Could you check a few things on this model? Use its own coordinates, in mm. A direction names the side the tool comes from. Give positions to 0.01 mm unless a question says otherwise; leave off trailing zeros. Loops run counter-clockwise (first coordinate to the right, second up) from the corner with the lowest first, then second, coordinate; pieces in that order, holes last. Notation, with made-up numbers: M 55.5,44.5 L 69.5,44.5 A24 ccw 69.5,60.5 Z; hole C 17,27 d7. An arc over 180 degrees is marked long. Use a Markdown table: item, result. Add a question column.
1) Suppose I cut it at C-C on y = 13.75. List the corners of the cut face in (x, z) for me.
2) Which directions (+Z, -Z, +X, -X, +Y, -Y) give clear straight access to the entire face, cutting with the end or side of a thin tool? Please do faces 4 (the flat face through (8, 9, 8)), 5 (the cylindrical face through (-12.04, 5.53, 20.46)), 6 (the flat face through (5, 11, 0)).
3) Suppose I cut it at B-B on z = 0. Count the separate pieces of the cut face and the enclosed holes in it, and give its area (3 significant figures).
4) Suppose I cut it at D-D on x = 26. List the corners of the cut face in (y, z) for me, and give its area (3 significant figures).
5) We'd pull the mould along X, two halves only. Please class faces 1 (the flat face through (-8, 11, 20)), 2 (the cylindrical face through (-32.19, 2.54, -32.84)), 3 (the flat face through (11, 8, 28)): +X half, -X half, draft (parallel to the pull), parting line (faces both ways), or undercut.
6) Will these pins go through, and if not, where does the flat tip stop? pin 1 Ø7 at (x, z) = (34, -34) entering from +Y; pin 2 Ø4 at (y, z) = (9, -10) entering from +X; pin 3 Ø3.5 at (y, z) = (9, -9.5) entering from -X.
7) Suppose I cut it at A-A on y = 1.25. List the corners of the cut face in (x, z) for me.
8) If I drill on line 1 along X through (y, z) = (11, 6.5); line 2 along Z through (x, y) = (5.8, 9); line 3 along X through (y, z) = (10.5, 18), over which ranges is the centre line in solid material (lowest first)? Write a range as [from, to].
```python
from build123d import *

# Parameters (mm, degrees)
SKETCH1_W           = 88
SKETCH1_H           = 88
BOSS_EXTRUDE1_DEPTH = 5
FILLET1_R           = 10
SKETCH2_R           = 2.15
CUT_EXTRUDE1_DEPTH  = 63.42595614
SKETCH3_W           = 4
SKETCH3_H           = 50
BOSS_EXTRUDE2_DEPTH = 10
CHAMFER1_SIZE       = 10
SKETCH4_R           = 1.5
CUT_EXTRUDE2_DEPTH  = 65.007812023
SKETCH5_R           = 3.5
CUT_EXTRUDE3_DEPTH  = 36
CUT_EXTRUDE4_START  = -36
SKETCH6_R           = 3.5
CUT_EXTRUDE4_DEPTH  = 36
LPATTERN2_COUNT     = 5
LPATTERN2_PITCH     = 10
CHAMFER2_SIZE       = 6


with BuildPart() as part:
    # Sketch1 → Boss-Extrude1 (new body)
    with BuildSketch(Plane(origin=(0, 0, 0), x_dir=(1, 0, 0), z_dir=(0, 1, 0))):
        Rectangle(SKETCH1_W, SKETCH1_H)
    extrude(amount=BOSS_EXTRUDE1_DEPTH)

    # Fillet1
    fillet1_edges = [part.edges().sort_by_distance(p)[0] for p in [
        (-44, 2.5, -44),
        (44, 2.5, -44),
        (44, 2.5, 44),
        (-44, 2.5, 44),
    ]]
    fillet(fillet1_edges, radius=FILLET1_R)

    # Sketch2 → Cut-Extrude1 (cut, through all)
    with BuildSketch(Plane(origin=(0, 5, 0), x_dir=(1, 0, 0), z_dir=(0, 1, 0))):
        with Locations(Location((34, 34, 0), (0, 0, 270))):
            Circle(SKETCH2_R)
        with Locations(Location((34, -34, 0), (0, 0, 270))):
            Circle(SKETCH2_R)
        with Locations(Location((-34, -34, 0), (0, 0, 270))):
            Circle(SKETCH2_R)
        with Locations(Location((-34, 34, 0), (0, 0, 270))):
            Circle(SKETCH2_R)
    extrude(amount=-CUT_EXTRUDE1_DEPTH, mode=Mode.SUBTRACT)

    # Sketch3 → Boss-Extrude2 (add)
    with BuildSketch(Plane(origin=(0, 5, 0), x_dir=(1, 0, 0), z_dir=(0, 1, 0))):
        with Locations((-7, 0)):
            Rectangle(SKETCH3_W, SKETCH3_H)
        with Locations((7, 0)):
            Rectangle(SKETCH3_W, SKETCH3_H)
    extrude(amount=BOSS_EXTRUDE2_DEPTH)

    # Chamfer1
    chamfer1_edges = [part.edges().sort_by_distance(p)[0] for p in [
        (9, 5, 0),
        (-9, 5, 0),
    ]]
    chamfer(chamfer1_edges, length=CHAMFER1_SIZE - 0.0001)  # a hair under: the kernel refuses the full size

    # Sketch4 → Cut-Extrude2 (cut, symmetric)
    with BuildSketch(Plane(origin=(0, 0, 0), x_dir=(0, 0, -1), z_dir=(1, 0, 0))):
        with Locations(Location((-20, 9, 0), (0, 0, 90))):
            Circle(SKETCH4_R)
    cut_extrude2 = extrude(amount=CUT_EXTRUDE2_DEPTH, both=True, mode=Mode.SUBTRACT)

    # Sketch5 → Cut-Extrude3 (cut)
    with BuildSketch(Plane(origin=(44, 0, 0), x_dir=(0, 0, -1), z_dir=(1, 0, 0))):
        with Locations((-20, 9)):
            Circle(SKETCH5_R)
    cut_extrude3 = extrude(amount=-CUT_EXTRUDE3_DEPTH, mode=Mode.SUBTRACT)

    # Sketch6 → Cut-Extrude4 (cut)
    with BuildSketch(Plane.ZY.offset(44).offset(CUT_EXTRUDE4_START)):
        with Locations(Location((20, 9, 0), (0, 0, 180))):
            Circle(SKETCH6_R)
    cut_extrude4 = extrude(amount=CUT_EXTRUDE4_DEPTH, mode=Mode.SUBTRACT)

    # LPattern2: Cut-Extrude2, Cut-Extrude3, Cut-Extrude4 ×5
    with Locations(*[(0, 0, -i * LPATTERN2_PITCH) for i in range(1, LPATTERN2_COUNT)]):
        add(cut_extrude2, mode=Mode.SUBTRACT)
        add(cut_extrude3, mode=Mode.SUBTRACT)
        add(cut_extrude4, mode=Mode.SUBTRACT)

    # Chamfer2
    chamfer2_edges = [part.edges().sort_by_distance(p)[0] for p in [
        (-11.99995, 5, -25),
        (-11.99995, 5, 25),
        (11.99995, 5, -25),
        (11.99995, 5, 25),
    ]]
    chamfer(chamfer2_edges, length=CHAMFER2_SIZE)


solid = part.part
```
Answer block:
| question | item | result |
|---|---|---|
| 1 | outline | M -10.25,-25 L -5,-25 L -5,25 L -10.25,25 Z; M 5,-25 L 10.25,-25 L 10.25,25 L 5,25 Z |
| 2 | face 4 | +X |
| 2 | face 5 | -X |
| 2 | face 6 | +Z, -Z, +Y |
| 3 | separate pieces | 3 |
| 3 | enclosed holes | 0 |
| 3 | area | 504 mm^2 |
| 4 | outline | M 0,-44 L 5,-44 L 5,44 L 0,44 Z |
| 4 | area | 440 mm^2 |
| 5 | face 1 | -X half |
| 5 | face 2 | undercut |
| 5 | face 3 | draft |
| 6 | pin 1 | stops at y = 5 |
| 6 | pin 2 | stops at x = 8 |
| 6 | pin 3 | stops at x = -8 |
| 7 | outline | M -44,-34 A10 ccw -34,-44 L 34,-44 A10 ccw 44,-34 L 44,34 A10 ccw 34,44 L -34,44 A10 ccw -44,34 Z; hole C -34,-34 d4.3; hole C -34,34 d4.3; hole C 34,-34 d4.3; hole C 34,34 d4.3 |
| 8 | line 1 | x = [-13, -5], [5, 13] |
| 8 | line 2 | z = [-27, -21.5], [-18.5, -11.5], [-8.5, -1.5], [1.5, 8.5], [11.5, 18.5], [21.5, 27] |
| 8 | line 3 | x = [-8, -5], [5, 8] |
